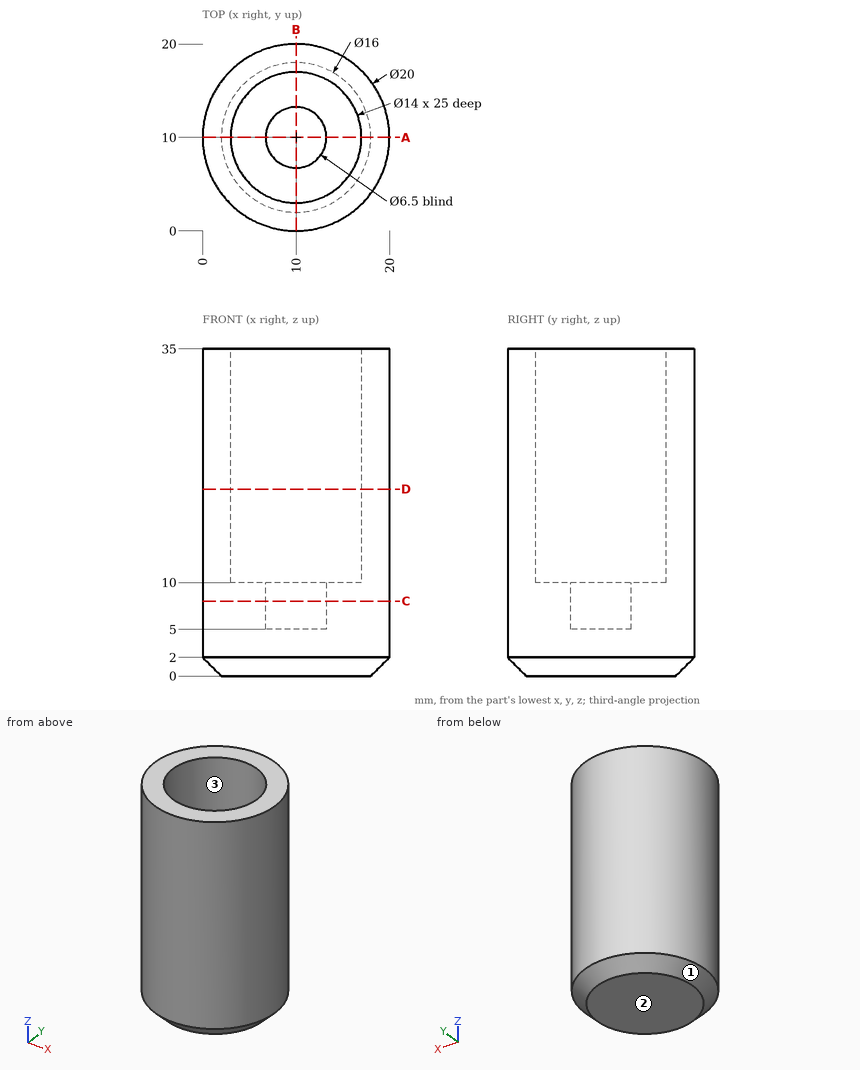
Study the drawing (mm; zero at the part's minimum x, y, z) and answer. Give positions to 0.01 mm unless a question says otherwise; leave off trailing zeros. Order: outer loops, then holes, each group sorted by start corner. A loop starts at its lowest first (then second) coordinate and runs counter-clockwise, first axis right, second up.
1) Find section D-D on z = 20. Write down the section's boundary in (x, y), then the cut area to 3 significant figures.
Reported:
outline: circle Ø20 at (10, 10); hole circle Ø14 at (10, 10)
area: 160 mm2
2) Given P1, Ø7, axis at x = 9.5, y = 10.5, coming from the +Z side; P2, Ø5, axis at x = 3.5, z = 29.5, coming from the +Y side; P3, Ø6, axis at x = 2.5, z = 10, coming from the +Y side, each flat-ended and moving along its own axis, determine where each tip first touches the part or whether it passes through.
Reported:
P1: stops at z = 10
P2: stops at y = 19.17
P3: stops at y = 18.93
3) Find section A-A on y = 10. Write down the section's boundary in (x, z).
Reported:
outline: (0, 2) - (2, 0) - (18, 0) - (20, 2) - (20, 35) - (17, 35) - (17, 10) - (13.25, 10) - (13.25, 5) - (6.75, 5) - (6.75, 10) - (3, 10) - (3, 35) - (0, 35) - close
4) Find section C-C on z = 8. Write down the section's boundary in (x, y).
Reported:
outline: circle Ø20 at (10, 10); hole circle Ø6.5 at (10, 10)
5) Consider line 1 along Y through (x, z) = (10, 15.5); line 2 along Y through (x, z) = (10, 6.8); line 3 along Z through (x, y) = (8.5, 8.25). Determine where each line is inside the solid, lowest interval first.
Reported:
line 1: y = 0 to 3, 17 to 20
line 2: y = 0 to 6.75, 13.25 to 20
line 3: z = 0 to 5
6) Determine the mould class of the marked faces 1, 2 and 3 for opening direction X: pulls with the +X half, pulls with the -X half, needs draft (parallel to the pull), parting line crosses it, or undercut.
Reported:
face 1: parting line crosses it
face 2: needs draft
face 3: undercut
